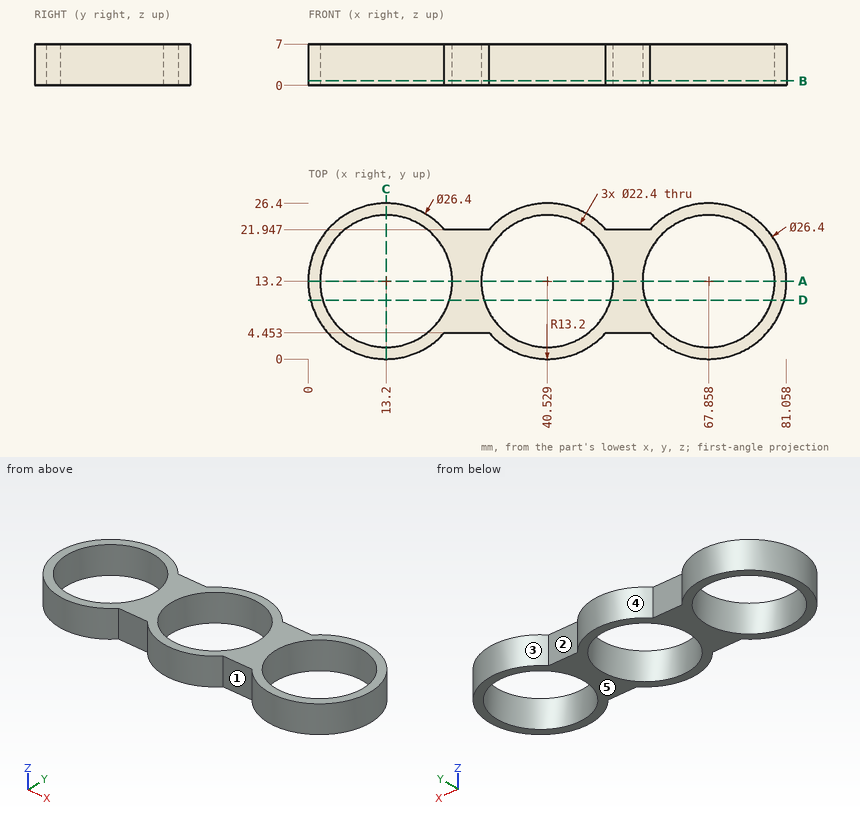
Geometry: see drawing. Coordinates: mm, zero at the bounding-box minimum. A direction names the side the tool comes from. Give positions to 0.01 mm unless a question says otherwise; leave off trailing zeros. Loops run counter-clockwise (first coordinate to the right, second up) from the corner with the lowest first, then second, coordinate; pieces in that order, holes last. Notation, with made-up numbers: M -27.75,26 L 15.25,26 A14 cw 15.25,39 Z; hole C 54,-21 d8. An arc over 180 degrees is marked long. Use one line per item in the form item = value.
1. Reachability of the marked faces 1, 2 and 3 from +Z, -Z, +X, -X, +Y, -Y: full face, straight path, thin tool, end or side. Return the list, or none.
Numbers:
face_1 = +Z, -Z, -Y
face_2 = +Z, -Z, +Y
face_3 = +Z, -Z
2. Pull-direction query (X, two-part tool) for the marked faces 4 and 5; classes: released by +X, released by -X, zero draft, split by the parting line, or undercut.
Numbers:
face_4 = undercut
face_5 = zero draft
3. Section query B-B, the plane z = 0.75. Return the cut outline in (x, y) (1 decimal).
Numbers:
outline = M 23.1,4.5 L 30.6,4.5 A13.2 ccw 50.4,4.5 L 58,4.5 A13.2 ccw long 58,21.9 L 50.4,21.9 A13.2 ccw 30.6,21.9 L 23.1,21.9 A13.2 ccw long Z; hole C 13.2,13.2 d22.4; hole C 40.5,13.2 d22.4; hole C 67.9,13.2 d22.4
4. First-contact query: pin 1 (3 mm diameter, centred on y = 11, z = 3, fed in from +X); pin 2 (3 mm diameter, centred on x = 58, y = 22.5, fed in from -Z); pin 3 (2 mm diameter, centred on y = 17.5, z = 5, fed in from -X); pin 4 (4 mm diameter, centred on x = 31.5, y = 13, fed in from -Z). Flat tips, straight axial feed; report the tip coordinate or a pass-through.
Numbers:
pin_1 = 81.04
pin_2 = 0
pin_3 = 0.42
pin_4 = through
5. Section query A-A, the plane y = 13.2. Return the cut outline in (x, z).
Numbers:
outline = M 0,0 L 2,0 L 2,7 L 0,7 Z; M 24.4,0 L 29.33,0 L 29.33,7 L 24.4,7 Z; M 51.73,0 L 56.66,0 L 56.66,7 L 51.73,7 Z; M 79.06,0 L 81.06,0 L 81.06,7 L 79.06,7 Z
6. Section query D-D, the plane y = 10. Return the cut outline in (x, z) (1 decimal), and give its area (3 significant figures).
Numbers:
outline = M 0.4,0 L 2.5,0 L 2.5,7 L 0.4,7 Z; M 23.9,0 L 29.8,0 L 29.8,7 L 23.9,7 Z; M 51.3,0 L 57.1,0 L 57.1,7 L 51.3,7 Z; M 78.6,0 L 80.7,0 L 80.7,7 L 78.6,7 Z
area = 111 mm²
7. Section query C-C, the plane x = 13.2. Return the cut outline in (y, z).
Numbers:
outline = M 0,0 L 2,0 L 2,7 L 0,7 Z; M 24.4,0 L 26.4,0 L 26.4,7 L 24.4,7 Z
8. Line query: L1, parallel to Y at x = 13.2, z = 3.75; L2, parallel to X at y = 15.5, z = 3; L3, parallel to X at y = 14, z = 3.5 (1 decimal). Output: solid intervals per line, ascending.
Numbers:
L1 = 0 to 2, 24.4 to 26.4
L2 = 0.2 to 2.24, 24.16 to 29.57, 51.49 to 56.9, 78.82 to 80.86
L3 = 0 to 2, 24.4 to 29.4, 51.7 to 56.7, 79 to 81
